from build123d import *

# Parameters (mm, degrees)
BOSS_EXTRUDE1_DEPTH = 166.124


with BuildPart() as part:
    # Sketch1 → Boss-Extrude1 (new body)
    with BuildSketch(Plane(origin=(0, 0, 0), x_dir=(0, 0, -1), z_dir=(1, 0, 0))):
        with BuildLine():
            Line((0, -20), (0, -5))
            ThreePointArc((0, -5), (1.464466094, -1.464466094), (5, 0))
            Line((5, 0), (20, 0))
            Line((20, 0), (20, -3.175))
            Line((20, -3.175), (47.585786438, -3.175))
            ThreePointArc((47.585786438, -3.175), (48.50966597, -3.792316568), (48.292893219, -4.882106781))
            Line((48.292893219, -4.882106781), (4.882106781, -48.292893219))
            ThreePointArc((4.882106781, -48.292893219), (3.792316568, -48.50966597), (3.175, -47.585786438))
            Line((3.175, -47.585786438), (3.175, -20))
            Line((3.175, -20), (0, -20))
        make_face()
    extrude(amount=BOSS_EXTRUDE1_DEPTH)


solid = part.part
Geometry: final body of the model. Coordinates: model frame, mm. A direction names the side the tool comes from. Give positions to 0.01 mm unless a question says otherwise; leave off trailing zeros. Loops run counter-clockwise (first coordinate to the right, second up) from the corner with the lowest first, then second, coordinate; pieces in that order, holes last. Notation, with made-up numbers: (-4, 3) - (43, 3) arc R6 cw to (43, 13) - close; hole circle Ø8 at (48, -1). An arc over 180 degrees is marked (long way). Answer as CSV lines item,"result". Start each with the question number.
1. Section C-C, the plane z = -25. Return loops of the section in (x, y) (3 decimals).
2. Reachability of faces 1 (the face through (82, -2, -20)), 2 (the face through (82, -20, -2)), 3 (the face through (82, -2, -1)) from +Z, -Z, +X, -X, +Y, -Y: full face, straight path, thin tool, end or side. Return the list, or none.
3. Section B-B, the plane y = -22.5. Return loops of the section in (x, z) (3 decimals).
4. Ray query, L1, parallel to Z at x = 128, y = -9.5 (3 decimals); L2, parallel to Z at x = 87, y = -25.5 (3 decimals); L3, parallel to Y at x = 129.5, z = -15.5 (3 decimals). Return the intervals inside material, ascending.
5. Section A-A, the plane x = 150.5. Return loops of the section in (y, z) (3 decimals).
6. Pin query (flat end, axial travel): P1, Ø12, axis at y = -32, z = -30, coming from the +X side; P2, Ø3, axis at x = 129.5, z = -27.5, coming from the +Y side (3 decimals); P3, Ø3.5, axis at x = 71.5, z = -1, coming from the -Y side; P4, Ø1, axis at x = 109, y = -16, coming from the -Z side (3 decimals). Return the tip coordinate at first contact, or that it passes through.
Answers:
1,outline,"(0, -28.175) - (166.124, -28.175) - (166.124, -3.175) - (0, -3.175) - close"
2,face 1,"-Z, +X, -X, +Y"
2,face 2,"+Z, +X, -X, -Y"
2,face 3,"+Z, +X, -X, +Y"
3,outline,"(0, -30.675) - (166.124, -30.675) - (166.124, -3.175) - (0, -3.175) - close"
4,L1,"z = -43.675 to 0"
4,L2,"z = -27.675 to -3.175"
4,L3,"y = -37.675 to 0"
5,outline,"(-48.293, -4.882) - (-4.882, -48.293) arc R1 ccw to (-3.175, -47.586) - (-3.175, -20) - (0, -20) - (0, -5) arc R5 ccw to (-5, 0) - (-20, 0) - (-20, -3.175) - (-47.586, -3.175) arc R1 ccw to start"
6,P1,"passes through"
6,P2,"stops at y = -3.175"
6,P3,"stops at y = -20"
6,P4,"stops at z = -37.675"
